Design review of the part built by this model. Coordinates are the model's own, in mm. A direction names the side the tool comes from. Give positions to 0.01 mm unless a question says otherwise; leave off trailing zeros. Write each loop counter-clockwise with the first axis right and the second up, starting at its lowest first coordinate (ties: lowest second). Pieces come first, ordered by that corner, then holes. Notation, with made-up numbers: M -18.5,11 L 29.5,11 A15 cw 29.5,38 Z; hole C 23.25,-30 d1. An arc over 180 degrees is marked long. Answer in a Markdown table with one row per item.
```python
from build123d import *

# Parameters (mm, degrees)
F0_W     = 10
F0_H     = 2
F1_DEPTH = 2
F2_W     = 2.41
F2_H     = 2
F3_DEPTH = 10.2
F4_DEPTH = 40


with BuildPart() as f1:
    # F0 (on Front) → F1 (new body)
    with BuildSketch(Plane.XZ):
        with Locations((6.96, 1)):
            Rectangle(F0_W, F0_H)
        with Locations((-6.96, 1)):
            Rectangle(F0_W, F0_H)
        with BuildLine():
            ThreePointArc((1.96, 0), (0, -1.96), (-1.96, 0))
            Line((-1.96, 0), (-11.96, 0))
            Line((-11.96, 0), (-11.96, -20))
            Line((-11.96, -20), (11.96, -20))
            Line((11.96, -20), (11.96, 0))
            Line((11.96, 0), (1.96, 0))
        make_face()
    extrude(amount=F1_DEPTH)

    # F2 (on Front) → F3 (join)
    with BuildSketch(Plane.XZ):
        with BuildLine():
            ThreePointArc((9.55, 0), (0, -9.55), (-9.55, 0))
            Line((-9.55, 0), (-11.96, 0))
            Line((-11.96, 0), (-11.96, -20))
            Line((-11.96, -20), (11.96, -20))
            Line((11.96, -20), (11.96, 0))
            Line((11.96, 0), (9.55, 0))
        make_face()
        with Locations((-10.755, 1)):
            Rectangle(F2_W, F2_H)
        with Locations((10.755, 1)):
            Rectangle(F2_W, F2_H)
    extrude(amount=-F3_DEPTH)

    # F0 (on Front) → F4 (join, symmetric)
    with BuildSketch(Plane.XZ):
        Polygon((11.96, -20), (-11.96, -20), (-36.96, -20), (-36.96, -22), (36.96, -22), (36.96, -20), align=None)
    extrude(amount=F4_DEPTH, both=True)


solid = f1.part
```
1) Add section B-B (z = -5). Write out the cut boundary in (x, y).
Geometry says:
| item | result |
|---|---|
| outline | M -11.96,-2 L 11.96,-2 L 11.96,10.2 L 8.14,10.2 L 8.14,0 L -8.14,0 L -8.14,10.2 L -11.96,10.2 Z |
2) Insertion check: P1, Ø3, axis at x = 11, y = 21.5, coming from the +Z side; P2, Ø11, axis at x = 3.5, z = -14, coming from the -Y side; P3, Ø12, axis at x = -13, z = -19, coming from the +Y side; P4, Ø1.6, axis at y = -1.5, z = 1, coming from the +X side. Each pin has a flat end and moves straight along its axis. Give the tip position at first contact, or say it passes through.
Geometry says:
| item | result |
|---|---|
| P1 | z = -20 |
| P2 | y = -2 |
| P3 | y = 40 |
| P4 | x = 11.96 |
3) To check wall thickness, follow probe 1 along Y at (x, z) = (0.5, -16); probe 2 along Z at (x, y) = (10.5, -18.5); probe 3 along X at (y, z) = (0, -12). State the ranges of each line that lie inside material, in increasing order. Write a range as [from, to].
Geometry says:
| item | result |
|---|---|
| probe 1 | [-2, 10.2] |
| probe 2 | [-22, -20] |
| probe 3 | [-11.96, 11.96] |
4) Add section D-D (x = 32.5). Write out the cut boundary in (y, z).
Geometry says:
| item | result |
|---|---|
| outline | M -40,-22 L 40,-22 L 40,-20 L -40,-20 Z |
5) Add section A-A (x = 0). Write out the cut boundary in (y, z).
Geometry says:
| item | result |
|---|---|
| outline | M -40,-22 L 40,-22 L 40,-20 L 10.2,-20 L 10.2,-9.55 L 0,-9.55 L 0,-1.96 L -2,-1.96 L -2,-20 L -40,-20 Z |
6) Add section C-C (y = 14.5). Write out the cut boundary in (x, z), and give its area (3 significant figures).
Geometry says:
| item | result |
|---|---|
| outline | M -36.96,-22 L 36.96,-22 L 36.96,-20 L -36.96,-20 Z |
| area | 148 mm^2 |
7) For faces 5 (the face through (-1.96, -1, 1)), 6 (the face through (0, -2, -9)), 7 (the face through (-11.96, 4, -9)), 8 (the face through (-9.55, 5, 1)), list the 3-axis set-ups (+Z, -Z, +X, -X, +Y, -Y) from which the entire face can be reached by the end or side of a thin tool; tool diameter is ignored.
Geometry says:
| item | result |
|---|---|
| face 5 | +Z, +Y, -Y |
| face 6 | +Z, +X, -X, -Y |
| face 7 | +Z, -X, +Y, -Y |
| face 8 | +Z, +Y |
8) The part is to be moulded in two halves that separate along X. For faces 1 (the face through (11.96, 4, -9)), 2 (the face through (-0.1, 0, -2.4)), 3 (the face through (0, 10.2, -11)), 4 (the face through (0.21, 5.029, -9.548)), say which applies: released by +X, released by -X, zero draft, split by the parting line, or undercut.
Geometry says:
| item | result |
|---|---|
| face 1 | released by +X |
| face 2 | undercut |
| face 3 | zero draft |
| face 4 | undercut |
